Check sheet for the drawn part. Datum: minimum x, y, z corner. Units: mm. Coordinates: 2 decimals unless noted, no trailing zeros. Order: outer loops, then holes, each group sorted by start corner. A loop starts at its lowest first (then second) coordinate and runs counter-clockwise, first axis right, second up.
Q1. Thickness scan on line 1 (Y direction, x = 4, z = 5); line 2 (X direction, y = 47, z = 7.5); line 3 (X direction, y = 12.5, z = 7.75). Record the ranges inside material, lowest first.
Q2. Cross-section at B-B, the plane z = 1.75. Record the boundary of the cut face in (x, y).
Q3. Cross-section at A-A, the plane y = 115.5. Record the boundary of the cut face in (x, z) (1 decimal).
Q4. Depth check by flat-ended pin: P1, Ø5, axis at x = 7, y = 61, coming from the -Z side; P2, Ø1.8, axis at x = 6, y = 76, coming from the +Z side; P3, Ø5, axis at x = 1.5, y = 72, coming from the -Z side. Enter the tip coordinate at first touch or a pass-through.
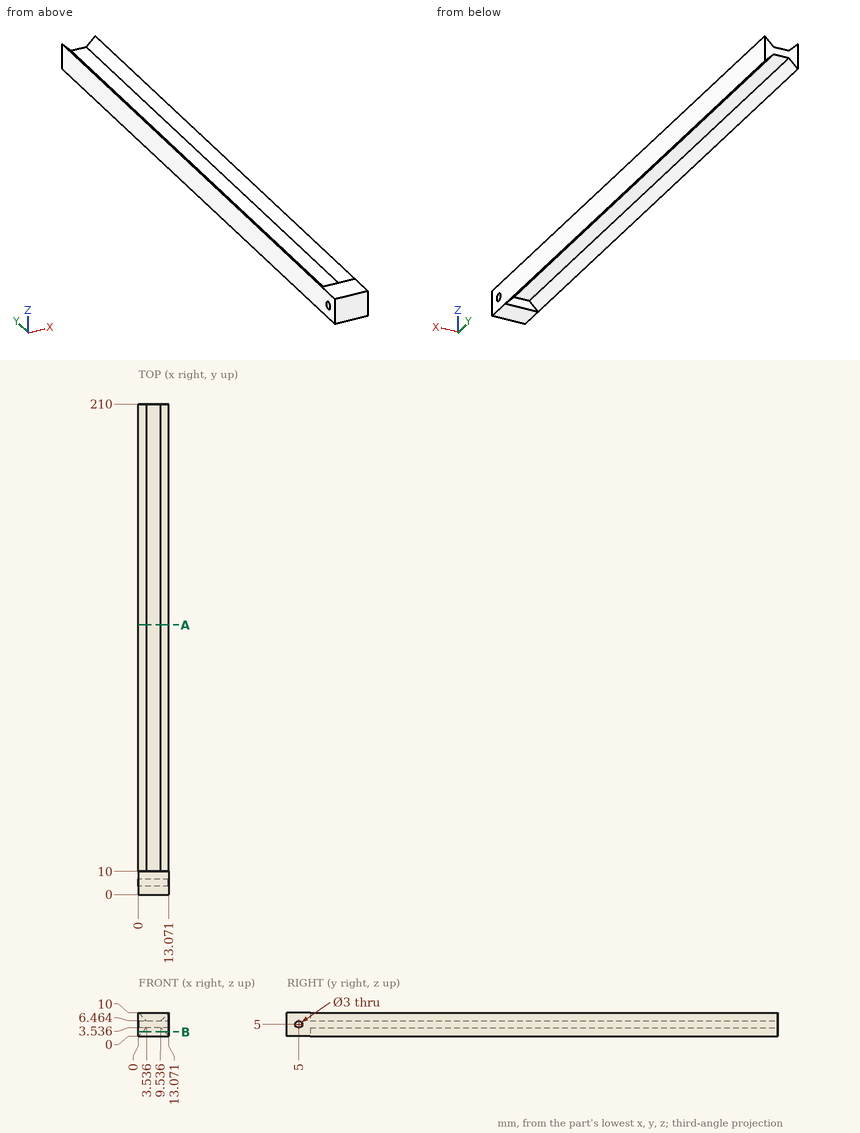
Check values:
1. line 1: y = 0 to 3.5, 6.5 to 210
1. line 2: x = 0 to 2.5, 10.57 to 13.07
1. line 3: x = 0 to 2.25, 10.82 to 13.07
2. outline: (0, 0) - (13.07, 0) - (13.07, 210) - (11.32, 210) - (11.32, 10) - (1.75, 10) - (1.75, 210) - (0, 210) - close
3. outline: (0, 0) - (3.5, 3.5) - (9.5, 3.5) - (13.1, 0) - (13.1, 10) - (9.5, 6.5) - (3.5, 6.5) - (0, 10) - close
4. P1: stops at z = 3.54
4. P2: stops at z = 6.46
4. P3: stops at z = 0
